```python
from build123d import *

# Parameters (mm, degrees)
SKETCH1_W         = 22.098
SKETCH1_H         = 22.098
EXTRUDE1_DEPTH    = 17.2212
FILLET1_R         = 0.635
SKETCH2_R         = 7.62
EXTRUDE2_DEPTH    = 7.112
EXTRUDE2_TAPER    = 1
SKETCH3_R         = 6.165117765
EXTRUDE3_DEPTH    = 7.7216
SKETCH4_R         = 6.985
EXTRUDE4_DEPTH    = 4.1402
SKETCH5_R         = 5.817229734
EXTRUDE5_DEPTH    = 3.683
DOME1_FACE_RADIUS = 5.817229734
DOME1_HEIGHT      = 3.683


with BuildPart() as part:
    # Sketch1 → Extrude1 (new body)
    with BuildSketch(Plane(origin=(0, 0, 0), x_dir=(1, 0, 0), z_dir=(0, 1, 0))):
        with Locations((11.049, 11.049)):
            Rectangle(SKETCH1_W, SKETCH1_H)
    extrude(amount=EXTRUDE1_DEPTH)

    # Fillet1
    fillet1_edges = [part.edges().sort_by_distance(p)[0] for p in [
        (22.098, 17.2212, -11.049),
        (11.049, 17.2212, -22.098),
        (0, 17.2212, -11.049),
        (11.049, 17.2212, 0),
        (0, 8.6106, -22.098),
        (22.098, 8.6106, -22.098),
        (22.098, 8.6106, 0),
        (0, 8.6106, 0),
    ]]
    fillet(fillet1_edges, radius=FILLET1_R)

    # Sketch2 → Extrude2 (add)
    with BuildSketch(Plane(origin=(0, 17.2212, 0), x_dir=(1, 0, 0), z_dir=(0, 1, 0))):
        with Locations((11.049, 11.049)):
            Circle(SKETCH2_R)
    extrude(amount=EXTRUDE2_DEPTH, taper=EXTRUDE2_TAPER)

    # Sketch3 → Extrude3 (add)
    with BuildSketch(Plane(origin=(0, 24.3332, 0), x_dir=(1, 0, 0), z_dir=(0, 1, 0))):
        with Locations((11.049, 11.049)):
            Circle(SKETCH3_R)
    extrude(amount=EXTRUDE3_DEPTH)

    # Sketch4 → Extrude4 (add)
    with BuildSketch(Plane(origin=(0, 32.0548, 0), x_dir=(1, 0, 0), z_dir=(0, 1, 0))):
        with Locations((11.049, 11.049)):
            Circle(SKETCH4_R)
    extrude(amount=EXTRUDE4_DEPTH)

    # Sketch5 → Extrude5 (cut)
    with BuildSketch(Plane(origin=(0, 36.195, 0), x_dir=(1, 0, 0), z_dir=(0, 1, 0))):
        with Locations((11.049, 11.049)):
            Circle(SKETCH5_R)
    extrude(amount=-EXTRUDE5_DEPTH, mode=Mode.SUBTRACT)

    # Dome1: a dome of height H over a round flat face of radius A is a cap of a sphere of radius (A * A + H * H) / (2 * H)
    dome1_r = (DOME1_FACE_RADIUS * DOME1_FACE_RADIUS + DOME1_HEIGHT * DOME1_HEIGHT) / (2 * DOME1_HEIGHT)
    dome1_base = Plane((11.049, 32.512, -11.049), z_dir=(0, 1, 0))
    with Locations(dome1_base.offset(DOME1_HEIGHT - dome1_r)):
        dome1_ball = Sphere(dome1_r, mode=Mode.PRIVATE)
    add(split(dome1_ball, bisect_by=dome1_base, keep=Keep.TOP, mode=Mode.PRIVATE))


solid = part.part
```
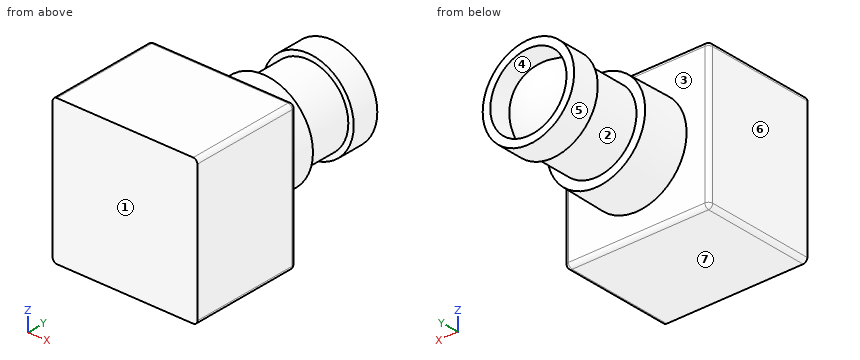
Design review of the part built by this model. Coordinates are the model's own, in mm. Face numbers are marked on the shaded views. A direction names the side the tool comes from. Give positions to 0.01 mm unless a question says otherwise; leave off trailing zeros. Write each loop counter-clockwise with the first axis right and the second up, starting at its lowest first coordinate (ties: lowest second). Pieces come first, ordered by that corner, then holes.
(1) Tool access review of the marked faces 1, 2 and 3: name each direction out of +Z, -Z, +X, -X, +Y, -Y from which nothing blocks a thin tool from reaching the whole face with its end or side.
Checked values:
face 1: +Z, -Z, +X, -X, -Y
face 2: none
face 3: +Y
(2) Add section B-B (z = -19.5). Give the boundary of the cut face in (x, y) (3 decimals), and give its area (3 significant figures).
Checked values:
outline: (0, 0) - (22.098, 0) - (22.098, 16.586) arc R0.635 ccw to (21.463, 17.221) - (0.635, 17.221) arc R0.635 ccw to (0, 16.586) - close
area: 380 mm2
(3) Add section C-C (y = 27). Give the boundary of the cut face in (x, z), and give its area (3 significant figures).
Checked values:
outline: circle Ø12.33 at (11.05, -11.05)
area: 119 mm2
(4) Add section D-D (y = 19). Give the boundary of the cut face in (x, z).
Checked values:
outline: circle Ø15.18 at (11.05, -11.05)
(5) Wall thickness on line 1 along Y through (x, z) = (5, -15); line 2 along Y through (x, z) = (16.75, -2); line 3 along X through (y, z) = (20, -13): over which ranges is each line inside the solid? List them lowest first.
Checked values:
line 1: y = 0 to 24.33
line 2: y = 0 to 17.22
line 3: x = 3.73 to 18.36
(6) Add section A-A (x = 20). Give the boundary of the cut face in (y, z) (3 decimals).
Checked values:
outline: (0, -22.098) - (16.586, -22.098) arc R0.635 ccw to (17.221, -21.463) - (17.221, -0.635) arc R0.635 ccw to (16.586, 0) - (0, 0) - close
(7) Mouldability with a two-part tool opening along Z and no side actions: class the marked faces 4, 5, 6 and 7 as +Z half, -Z half, draft (parallel to the pull), parting line (faces both ways), or undercut.
Checked values:
face 4: undercut
face 5: parting line
face 6: draft
face 7: -Z half
(8) Clearance check with flat-ended pins moving along their axes: pin 1 Ø1 at (y, z) = (29, -19) entering from -X; pin 2 Ø5 at (y, z) = (32, -14) entering from +X; pin 3 Ø4 at (x, z) = (19.5, -4) entering from +Y; pin 4 Ø5 at (x, z) = (13.5, -9) entering from +Y. State where each tip first meets the part, or that it passes through.
Checked values:
pin 1: passes through
pin 2: stops at x = 18.02
pin 3: stops at y = 17.22
pin 4: stops at y = 36.16
